Here's how the part is built. I have some questions about the finished solid (model axes, mm). Coordinates: 2 decimals unless noted, no trailing zeros. Order: outer loops, then holes, each group sorted by start corner. A loop starts at its lowest first (then second) coordinate and runs counter-clockwise, first axis right, second up. Notation, with made-up numbers: (-37, 83) - (12, 83) arc R28 ccw to (12, 102) - close; hole circle Ø5 at (-22.5, 72.25). An arc over 180 degrees is marked (long way). Use CSV: the item, a comma, the result in double quotes. Start each with the question number.
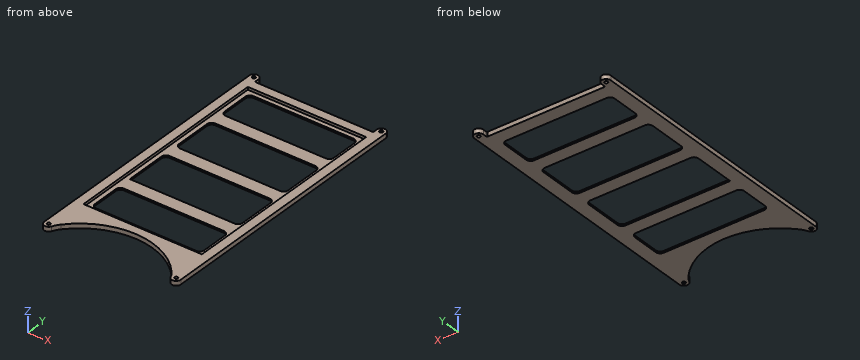
from build123d import *

# Parameters (mm, degrees)
SKETCH_2_R          = 1.8
EXTRUDE_1_DEPTH     = 5
SKETCH_3_W          = 130
SKETCH_3_H          = 234
CUT_EXTRUDE_1_DEPTH = 3
CUT_EXTRUDE_2_DEPTH = 302.492951825


with BuildPart() as part:
    # Эскиз2 → Бобышка-Вытянуть1 (new body)
    with BuildSketch(Plane.XY):
        with BuildLine():
            Line((-65, 5), (-65, 1))
            ThreePointArc((-65, 1), (-64.707106781, 0.292893219), (-64, 0))
            Line((-64, 0), (64, 0))
            ThreePointArc((64, 0), (64.707106781, 0.292893219), (65, 1))
            Line((65, 1), (65, 5))
            ThreePointArc((65, 5), (70, 10), (75, 5))
            Line((75, 5), (75, -287))
            ThreePointArc((75, -287), (71.029305531, -291.892906102), (65.42378795, -289.014518125))
            ThreePointArc((65.42378795, -289.014518125), (63.358638237, -285.125391065), (60.746425043, -281.58046584))
            ThreePointArc((60.746425043, -281.58046584), (0, -253.636895265), (-60.746425043, -281.58046584))
            ThreePointArc((-60.746425043, -281.58046584), (-63.358638237, -285.125391065), (-65.42378795, -289.014518125))
            ThreePointArc((-65.42378795, -289.014518125), (-71.029305531, -291.892906102), (-75, -287))
            Line((-75, -287), (-75, 5))
            ThreePointArc((-75, 5), (-70, 10), (-65, 5))
        make_face()
        with Locations((70, -287)):
            Circle(SKETCH_2_R, mode=Mode.SUBTRACT)
        with Locations((-70, -287)):
            Circle(SKETCH_2_R, mode=Mode.SUBTRACT)
        with Locations((-70, 5)):
            Circle(SKETCH_2_R, mode=Mode.SUBTRACT)
        with Locations((70, 5)):
            Circle(SKETCH_2_R, mode=Mode.SUBTRACT)
    extrude(amount=EXTRUDE_1_DEPTH)

    # Эскиз3 → Вырез-Вытянуть1 (cut)
    with BuildSketch(Plane.XY.offset(5)):
        with Locations((0, -127)):
            Rectangle(SKETCH_3_W, SKETCH_3_H)
    extrude(amount=-CUT_EXTRUDE_1_DEPTH, mode=Mode.SUBTRACT)

    # Эскиз4 → Вырез-Вытянуть2 (cut, through all)
    with BuildSketch(Plane.XY.offset(2)):
        with BuildLine():
            Line((-55, -15), (55, -15))
            ThreePointArc((55, -15), (58.535533906, -16.464466094), (60, -20))
            Line((60, -20), (60, -49.5))
            ThreePointArc((60, -49.5), (58.535533906, -53.035533906), (55, -54.5))
            Line((55, -54.5), (-55, -54.5))
            ThreePointArc((-55, -54.5), (-58.535533906, -53.035533906), (-60, -49.5))
            Line((-60, -49.5), (-60, -20))
            ThreePointArc((-60, -20), (-58.535533906, -16.464466094), (-55, -15))
        make_face()
        with BuildLine():
            Line((-55, -239), (55, -239))
            ThreePointArc((55, -239), (58.535533906, -237.535533906), (60, -234))
            Line((60, -234), (60, -204.5))
            ThreePointArc((60, -204.5), (58.535533906, -200.964466094), (55, -199.5))
            Line((55, -199.5), (-55, -199.5))
            ThreePointArc((-55, -199.5), (-58.535533906, -200.964466094), (-60, -204.5))
            Line((-60, -204.5), (-60, -234))
            ThreePointArc((-60, -234), (-58.535533906, -237.535533906), (-55, -239))
        make_face()
        with BuildLine():
            Line((55, -119.5), (-55, -119.5))
            ThreePointArc((-55, -119.5), (-58.535533906, -118.035533906), (-60, -114.5))
            Line((-60, -114.5), (-60, -74.5))
            ThreePointArc((-60, -74.5), (-58.535533906, -70.964466094), (-55, -69.5))
            Line((-55, -69.5), (55, -69.5))
            ThreePointArc((55, -69.5), (58.535533906, -70.964466094), (60, -74.5))
            Line((60, -74.5), (60, -114.5))
            ThreePointArc((60, -114.5), (58.535533906, -118.035533906), (55, -119.5))
        make_face()
        with BuildLine():
            Line((-60, -139.5), (-60, -184.5))
            Line((-60, -184.5), (55, -184.5))
            ThreePointArc((55, -184.5), (58.535533906, -183.035533906), (60, -179.5))
            Line((60, -179.5), (60, -139.5))
            ThreePointArc((60, -139.5), (58.535533906, -135.964466094), (55, -134.5))
            Line((55, -134.5), (-55, -134.5))
            ThreePointArc((-55, -134.5), (-58.535533906, -135.964466094), (-60, -139.5))
        make_face()
    extrude(amount=-CUT_EXTRUDE_2_DEPTH, mode=Mode.SUBTRACT)


solid = part.part
Item 1: Please list where these lines run through material, in increasing order: line 1 along Y through (x, z) = (70, 1.2); line 2 along X through (y, z) = (-39.5, 0.3); line 3 along X through (y, z) = (-287, 2.25). Write a range as from..to.
Item 2: Suppose I cut it at D-D on y = -271. Write out the boundary of the cut face in (x, z), then the cut area to 3 significant figures.
Item 3: For pin 1 Ø2 at (x, z) = (-15, 1.5) entering from +Y; pin 2 Ø3 at (x, y) = (-70, 5) entering from -Z; pin 3 Ø4 at (x, y) = (-70, -287) entering from -Z, each with a flat end and sliding along its axis, tell me the tip position at first contact or that it passes through.
Item 4: Suppose I cut it at C-C on x = -12. Write out the boundary of the cut face in (y, z), then the cut area to 3 significant figures.
Item 5: Suppose I cut it at B-B on z = 3.8. Write out the boundary of the cut face in (x, y), then the cut area to 3 significant figures.
Item 6: Suppose I cut it at A-A on y = -153. Write out the boundary of the cut face in (x, z), then the cut area to 3 significant figures.
Here are the results:
1,line 1,"-292..-288.8, -285.2..3.2, 6.8..10"
1,line 2,"-75..-60, 60..75"
1,line 3,"-75..-71.8, -68.2..-64.45, 64.45..68.2, 71.8..75"
2,outline,"(-75, 0) - (-49.77, 0) - (-49.77, 5) - (-75, 5) - close; (49.77, 0) - (75, 0) - (75, 5) - (49.77, 5) - close"
2,area,"252 mm^2"
3,pin 1,"y = 0"
3,pin 2,"through"
3,pin 3,"z = 0"
4,outline,"(-254.54, 0) - (-239, 0) - (-239, 2) - (-244, 2) - (-244, 5) - (-254.54, 5) - close; (-199.5, 0) - (-184.5, 0) - (-184.5, 2) - (-199.5, 2) - close; (-134.5, 0) - (-119.5, 0) - (-119.5, 2) - (-134.5, 2) - close; (-69.5, 0) - (-54.5, 0) - (-54.5, 2) - (-69.5, 2) - close; (-15, 0) - (0, 0) - (0, 5) - (-10, 5) - (-10, 2) - (-15, 2) - close"
4,area,"213 mm^2"
5,outline,"(-75, -287) arc R5 ccw to (-65.42, -289.01) arc R30 cw to (-60.75, -281.58) arc R80 cw to (60.75, -281.58) arc R30 cw to (65.42, -289.01) arc R5 ccw to (75, -287) - (75, 5) arc R5 ccw to (65, 5) - (65, 1) arc R1 cw to (64, 0) - (-64, 0) arc R1 cw to (-65, 1) - (-65, 5) arc R5 ccw to (-75, 5) - close; hole circle Ø3.6 at (-70, -287); hole circle Ø3.6 at (-70, 5); hole (-65, -244) - (65, -244) - (65, -10) - (-65, -10) - close; hole circle Ø3.6 at (70, -287); hole circle Ø3.6 at (70, 5)"
5,area,"9,810 mm^2"
6,outline,"(-75, 0) - (-60, 0) - (-60, 2) - (-65, 2) - (-65, 5) - (-75, 5) - close; (60, 0) - (75, 0) - (75, 5) - (65, 5) - (65, 2) - (60, 2) - close"
6,area,"120 mm^2"
